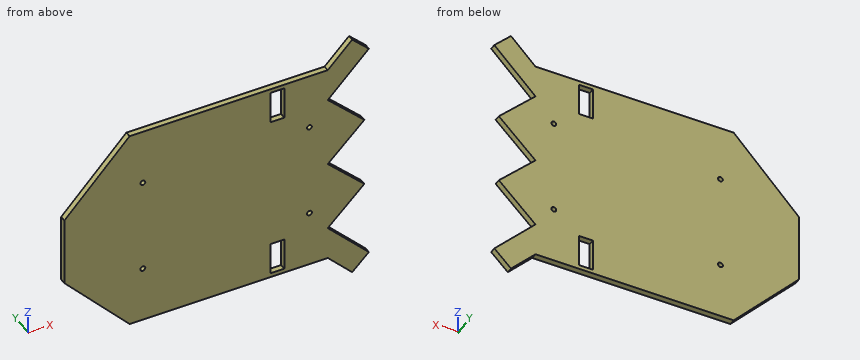
```python
from build123d import *

# Parameters (mm, degrees)
BOSS_EXTRUDE2_DEPTH      = 5
BOSS_EXTRUDE2_DEPTH_BACK = 0.1
SKETCH6_R                = 2.1
CUT_EXTRUDE2_DEPTH       = 10
SKETCH2_W                = 12
SKETCH2_H                = 28
CUT_EXTRUDE3_DEPTH       = 10


with BuildPart() as part:
    # Sketch1 → Boss-Extrude2 (new, two sides: drawn at the far end of the back side and taken through both)
    with BuildSketch(Plane(origin=(0, 0, 0), x_dir=(1, 0, 0), z_dir=(0, 1, 0)).offset(-BOSS_EXTRUDE2_DEPTH_BACK)):
        Polygon((0, -30), (0, 30), (55.94480687, 90), (225.94480687, 90), (246.912660032, 111.45574827), (261.216492211, 97.477179495), (225.94480687, 61.384767177), (257.353801996, 30.69), (225.94480687, 0), (257.353801996, -30.69), (225.94480687, -61.384767177), (261.216492211, -97.477179495), (246.912660032, -111.45574827), (225.94480687, -90), (55.94480687, -90), align=None)
    extrude(amount=BOSS_EXTRUDE2_DEPTH + BOSS_EXTRUDE2_DEPTH_BACK)

    # Sketch6 → Cut-Extrude2 (cut)
    with BuildSketch(Plane(origin=(0, -0.1, 0), x_dir=(-1, 0, 0), z_dir=(0, -1, 0))):
        with Locations(Location((-67.309752753, 41.081967218, 0), (0, 0, 90))):
            Circle(SKETCH6_R)
        with Locations(Location((-210.227358504, 41.081967218, 0), (0, 0, 90))):
            Circle(SKETCH6_R)
        with Locations(Location((-210.227358504, -41.081967218, 0), (0, 0, 270))):
            Circle(SKETCH6_R)
        with Locations(Location((-67.309752753, -41.081967218, 0), (0, 0, 270))):
            Circle(SKETCH6_R)
    extrude(amount=-CUT_EXTRUDE2_DEPTH, mode=Mode.SUBTRACT)

    # Sketch2 → Cut-Extrude3 (cut)
    with BuildSketch(Plane.XZ.offset(0.1)):
        with Locations((182.674603171, -72.444256033)):
            Rectangle(SKETCH2_W, SKETCH2_H)
        with Locations((182.674603171, 72.444256033)):
            Rectangle(SKETCH2_W, SKETCH2_H)
    extrude(amount=-CUT_EXTRUDE3_DEPTH, mode=Mode.SUBTRACT)


solid = part.part
```
Design review of the part built by this model. Coordinates are the model's own, in mm. Coordinates: 2 decimals unless noted, no trailing zeros. Write each loop counter-clockwise with the first axis right and the second up, starting at its lowest first coordinate (ties: lowest second). Pieces come first, ordered by that corner, then holes.
1) To check wall thickness, follow L1, parallel to Z at x = 246.5, y = 2.7; L2, parallel to Z at x = 249, y = 0.75; L3, parallel to X at y = 1.75, z = 74. State the ranges of each line that lie inside material, in increasing order.
2) Add section D-D (z = -83). Write out the cut boundary in (x, y).
3) Add section C-C (x = 166). Write out the cut boundary in (y, z).
4) Insertion check: pin 1 (1.5 mm diameter, centred on x = 181, y = 3.5, fed in from +Z); pin 2 (5 mm diameter, centred on x = 67.31, z = -41.08, fed in from +Y); pin 3 (4 mm diameter, centred on x = 210.23, z = 41.08, fed in from +Y); pin 4 (3 mm diameter, centred on y = 4, z = 76, fed in from +X). Each pin has a flat end and moves straight along its axis. Give the tip position at first contact, or say it passes through.
5) Add section B-B (y = 3.9). Write out the cut boundary in (x, z).
6) Add section A-A (z = 79). Write out the cut boundary in (x, y), plus the area to 3 significant figures.
Check result:
1. L1: z = -111.03 to -82.42, -41.3 to -20.08, 20.08 to 41.3, 82.42 to 111.03
1. L2: z = -109.42 to -84.98, -38.85 to -22.53, 22.53 to 38.85, 84.98 to 109.42
1. L3: x = 41.03 to 176.67, 188.67 to 238.27
2. outline: (49.42, -0.1) - (176.67, -0.1) - (176.67, 5) - (49.42, 5) - close; (188.67, -0.1) - (247.07, -0.1) - (247.07, 5) - (188.67, 5) - close
3. outline: (-0.1, -90) - (5, -90) - (5, 90) - (-0.1, 90) - close
4. pin 1: stops at z = 90
4. pin 2: stops at y = 5
4. pin 3: passes through
4. pin 4: stops at x = 241.69
5. outline: (0, -30) - (55.94, -90) - (225.94, -90) - (246.91, -111.46) - (261.22, -97.48) - (225.94, -61.38) - (257.35, -30.69) - (225.94, 0) - (257.35, 30.69) - (225.94, 61.38) - (261.22, 97.48) - (246.91, 111.46) - (225.94, 90) - (55.94, 90) - (0, 30) - close; hole circle Ø4.2 at (67.31, -41.08); hole circle Ø4.2 at (67.31, 41.08); hole (176.67, -86.44) - (188.67, -86.44) - (188.67, -58.44) - (176.67, -58.44) - close; hole (176.67, 58.44) - (188.67, 58.44) - (188.67, 86.44) - (176.67, 86.44) - close; hole circle Ø4.2 at (210.23, -41.08); hole circle Ø4.2 at (210.23, 41.08)
6. outline: (45.69, -0.1) - (176.67, -0.1) - (176.67, 5) - (45.69, 5) - close; (188.67, -0.1) - (243.16, -0.1) - (243.16, 5) - (188.67, 5) - close
6. area: 946 mm2
